For this review, take the finished solid that the model builds, in its own axes (mm). A direction names the side the tool comes from. Give positions to 0.01 mm unless a question says otherwise; leave off trailing zeros. Order: outer loops, then holes, each group sorted by start corner. A loop starts at its lowest first (then second) coordinate and runs counter-clockwise, first axis right, second up.
from build123d import *

# Parameters (mm, degrees)
F0_W      = 76.6343446126
F0_H      = 33.6732733995
F1_DEPTH  = 27.432
F2_SIZE   = 25.4
F3_SIZE   = 20.32
F4_W      = 3.1658643857
F4_H      = 24.8281476088
F5_DEPTH  = 25.4
F6_W      = 3.4536682069
F6_H      = 24.4211279787
F7_DEPTH  = 25.4
F8_W      = 3.4536719322
F8_H      = 24.4211279787
F9_DEPTH  = 25.4
F10_W     = 3.4536686726
F10_H     = 24.4211279787
F11_DEPTH = 25.4


with BuildPart() as f1:
    # F0 (on Front) → F1 (new body)
    with BuildSketch(Plane.XZ):
        Rectangle(F0_W, F0_H)
    extrude(amount=F1_DEPTH)

    # F2
    f2_edges = [f1.edges().sort_by_distance(p)[0] for p in [
        (0, -27.432, 16.836637),
    ]]
    chamfer(f2_edges, length=F2_SIZE)

    # F3
    f3_edges = [f1.edges().sort_by_distance(p)[0] for p in [
        (-38.317172, -14.732, 4.136637),
        (38.317172, -14.732, 4.136637),
    ]]
    chamfer(f3_edges, length=F3_SIZE)

    # F4 (on face) → F5 (cut)
    with BuildSketch(Plane(origin=(0, -9.4343183499, 9.4343183499), x_dir=(1, 0, 0), z_dir=(0, -0.7071067812, 0.7071067812))):
        with Locations((-12.0878419839, -7.6438782271)):
            Rectangle(F4_W, F4_H)
    extrude(amount=-F5_DEPTH, mode=Mode.SUBTRACT)

    # F6 (on face) → F7 (cut)
    with BuildSketch(Plane(origin=(0, -9.4343183499, 9.4343183499), x_dir=(1, 0, 0), z_dir=(0, -0.7071067812, 0.7071067812))):
        with Locations((-5.7953335345, -7.4403684121)):
            Rectangle(F6_W, F6_H)
    extrude(amount=-F7_DEPTH, mode=Mode.SUBTRACT)

    # F8 (on face) → F9 (cut)
    with BuildSketch(Plane(origin=(0, -9.4343183499, 9.4343183499), x_dir=(1, 0, 0), z_dir=(0, -0.7071067812, 0.7071067812))):
        with Locations((12.6242348924, -7.4403684121)):
            Rectangle(F8_W, F8_H)
    extrude(amount=-F9_DEPTH, mode=Mode.SUBTRACT)

    # F10 (on face) → F11 (cut)
    with BuildSketch(Plane(origin=(0, -9.4343183499, 9.4343183499), x_dir=(1, 0, 0), z_dir=(0, -0.7071067812, 0.7071067812))):
        with Locations((5.7168968488, -7.4403684121)):
            Rectangle(F10_W, F10_H)
    extrude(amount=-F11_DEPTH, mode=Mode.SUBTRACT)


solid = f1.part
1) We need section B-B on z = 4.5. Give the boundary of the cut face in (x, y), then the cut area to 3 significant figures.
Answer sheet:
outline: (-28.16, 0) - (-18, -14.37) - (-13.67, -14.37) - (-13.67, 0) - close; (-10.5, -14.37) - (-7.52, -14.37) - (-7.52, 0) - (-10.5, 0) - close; (-4.07, -14.37) - (3.99, -14.37) - (3.99, 0) - (-4.07, 0) - close; (7.44, -14.37) - (10.9, -14.37) - (10.9, 0) - (7.44, 0) - close; (14.35, -14.37) - (18, -14.37) - (28.16, 0) - (14.35, 0) - close
area: 469 mm2
2) We need section A-A on x = -5. Give the boundary of the cut face in (y, z).
Answer sheet:
outline: (-27.43, -16.84) - (-10.95, -16.84) - (-23.33, -4.46) - (-27.43, -8.56) - close; (-6.06, 12.81) - (0, 6.75) - (0, 16.84) - (-2.03, 16.84) - close
3) We need section D-D on z = -12.5. Give the boundary of the cut face in (x, y).
Answer sheet:
outline: (-38.32, -2.63) - (-20.78, -27.43) - (20.78, -27.43) - (38.32, -2.63) - (38.32, 0) - (14.35, 0) - (14.35, -15.29) - (10.9, -15.29) - (10.9, 0) - (7.44, 0) - (7.44, -15.29) - (3.99, -15.29) - (3.99, 0) - (-4.07, 0) - (-4.07, -15.29) - (-7.52, -15.29) - (-7.52, 0) - (-10.5, 0) - (-10.5, -15.87) - (-13.67, -15.87) - (-13.67, 0) - (-38.32, 0) - close
4) Clearance check with flat-ended pins moving along their axes: pin 1 (11.5 mm diameter, centred on y = -12.5, z = 5, fed in from -X); pin 2 (7 mm diameter, centred on y = -14.5, z = -6.5, fed in from +X); pin 3 (11.5 mm diameter, centred on y = -16, z = 4, fed in from -X). State where each tip first meets the part, or that it passes through.
Answer sheet:
pin 1: stops at x = -24.71
pin 2: stops at x = 29.18
pin 3: stops at x = -22.95
5) Draft analysis for pull direction X (two halves, no side actions). For faces 4 (the face through (0, -27.432, -13)), 5 (the face through (-38.317, -3, -14)), 6 (the face through (5.69, -17.23, -10.56)), state which applies: +X half, -X half, draft (parallel to the pull), parting line (faces both ways), or undercut.
Answer sheet:
face 4: draft
face 5: -X half
face 6: undercut
6) We need section C-C on y = -7.75. Give the boundary of the cut face in (x, z).
Answer sheet:
outline: (-37.76, -16.84) - (-13.67, -16.84) - (-13.67, 11.12) - (-18, 11.12) - close; (-10.5, -16.84) - (-7.52, -16.84) - (-7.52, 11.12) - (-10.5, 11.12) - close; (-4.07, -16.84) - (3.99, -16.84) - (3.99, 11.12) - (-4.07, 11.12) - close; (7.44, -16.84) - (10.9, -16.84) - (10.9, 11.12) - (7.44, 11.12) - close; (14.35, -16.84) - (37.76, -16.84) - (18, 11.12) - (14.35, 11.12) - close
7) To check wall thickness, follow line 1 (X direction, y = -9, z = 3); line 2 (X direction, y = -17.5, z = 0); line 3 (Z direction, x = -26.5, y = -20.5). State the ranges of each line that lie inside material, in increasing order.
Answer sheet:
line 1: x = -22.85 to -13.67, -10.5 to -7.52, -4.07 to 3.99, 7.44 to 10.9, 14.35 to 22.85
line 2: x = -18.96 to -13.67, -10.5 to -7.52, -4.07 to 3.99, 7.44 to 10.9, 14.35 to 18.96
line 3: z = -16.84 to -13.66
8) Tool access review of faces 1 (the face through (-25.76, -10.59, -2.7)), 2 (the face through (12.6, -17.23, -10.56)), 3 (the face through (12.6, -3.073, 9.819)): name each direction out of +Z, -Z, +X, -X, +Y, -Y from which nothing blocks a thin tool from reaching the whole face with its end or side.
Answer sheet:
face 1: +Z, -X, -Y
face 2: +Z, +Y
face 3: -Z, -Y
